Input: dimensioned drawing with shaded views. Units: mm. Origin: part minimum x, y, z. A direction names the side the tool comes from. Give positions to 0.01 mm unless a question says otherwise; leave off trailing zeros.
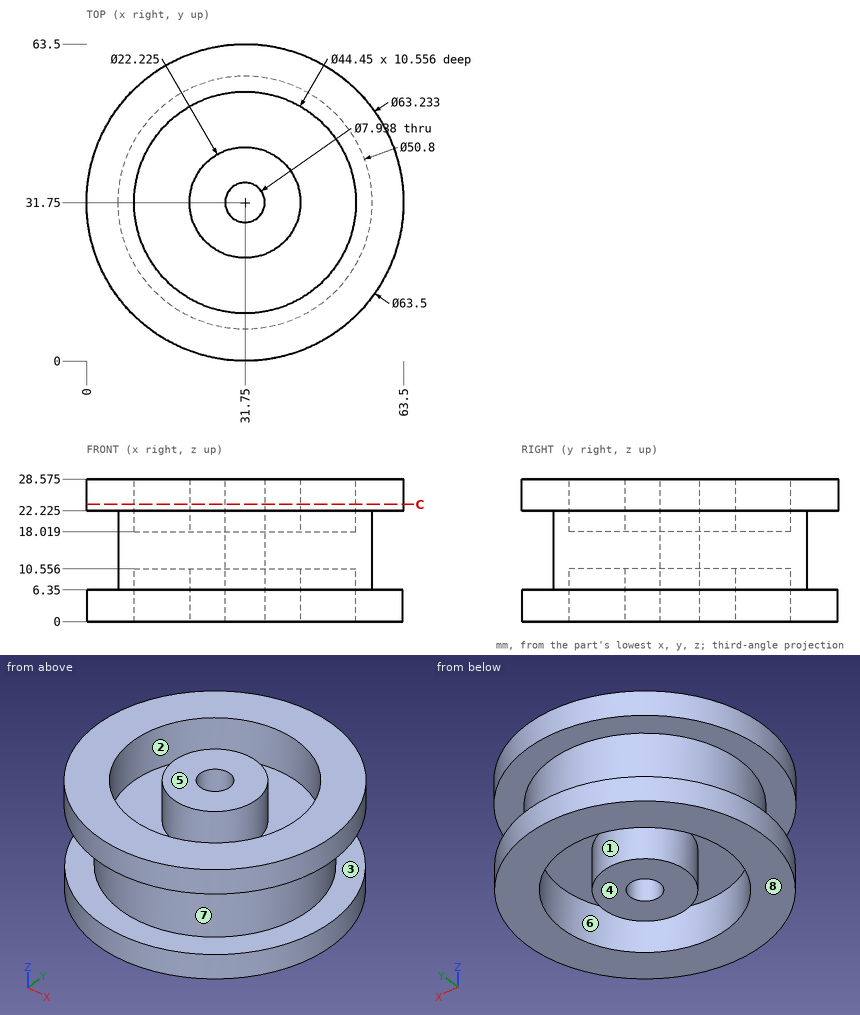
Item 1: Pin query (flat end, axial travel): pin 1 Ø6.5 at (x, y) = (31.75, 31.75) entering from +Z; pin 2 Ø3 at (x, z) = (41.5, 4.5) entering from -Y; pin 3 Ø3 at (y, z) = (19, 10.5) entering from +X; pin 4 Ø10 at (y, z) = (46.5, 11.5) entering from +X (1 decimal). Return the tip coordinate at first contact, or that it passes through.
Found:
pin 1: passes through
pin 2: stops at y = 1.23
pin 3: stops at x = 54.52
pin 4: stops at x = 55.2
Item 2: Reachability of the marked faces 1, 2, 3, 4 and 5 from +Z, -Z, +X, -X, +Y, -Y: full face, straight path, thin tool, end or side. Return the list, or none.
Found:
face 1: -Z
face 2: +Z
face 3: none
face 4: -Z, +X, -X, +Y, -Y
face 5: +Z, +X, -X, +Y, -Y
Item 3: Line query: L1, parallel to Y at x = 31.75, z = 3.5 (1 decimal); L2, parallel to Y at x = 31.75, z = 24.5 (1 decimal); L3, parallel to Y at x = 40, z = 24.25 (1 decimal). Output: solid intervals per line, ascending.
Found:
L1: y = 0.1 to 9.5, 20.6 to 27.8, 35.7 to 42.9, 54 to 63.4
L2: y = 0 to 9.5, 20.6 to 27.8, 35.7 to 42.9, 54 to 63.5
L3: y = 1.1 to 11.1, 24.3 to 39.2, 52.4 to 62.4
Item 4: Section C-C, the plane z = 23.5. State how many separate pieces and enclosed holes the cut face has, plus the area to 3 significant figures.
Found:
separate pieces: 2
enclosed holes: 2
area: 1,950 mm2
Item 5: Pull-direction query (Z, two-part tool) for the marked faces 6, 7 and 8; classes: +Z half, -Z half, draft (parallel to the pull), parting line (faces both ways), or undercut.
Found:
face 6: draft
face 7: undercut
face 8: -Z half
